Input: dimensioned drawing with shaded views. Units: mm. Origin: part minimum x, y, z. A direction names the side the tool comes from. Coordinates: 2 decimals unless noted, no trailing zeros. Order: outer loops, then holes, each group sorted by start corner. A loop starts at its lowest first (then second) coordinate and runs counter-clockwise, first axis right, second up. Notation, with made-up numbers: M -11,42.25 L 10,42.25 A32 ccw 10,78.25 Z; hole C 57.5,27.5 d6. An arc over 180 degrees is marked long. Use CSV: the item, a comma, the result in double quotes. Start each with the question number.
1. Pull-direction query (Y, two-part tool) for the marked faces 5, 6, 7 and 8; classes: pulls with the +Y half, pulls with the -Y half, needs draft (parallel to the pull), parting line crosses it, or undercut.
2. First-contact query: P1, Ø1.5, axis at y = 14.5, z = 37.5, coming from the -X side; P2, Ø3, axis at y = 3, z = 35, coming from the +X side; P3, Ø5, axis at y = 12.5, z = 54.5, coming from the +X side. Flat tips, straight axial feed; report the tip coordinate or a pass-through.
3. Section query C-C on z = 19. Return the cut outline in (x, y).
4. Section query B-B on x = 21. Return the cut outline in (y, z).
5. Material intervals for line 1 (Y direction, x = 24, z = 43.5); line 2 (Z direction, x = 25, y = 16.75); line 3 (X direction, y = 9.5, z = 5.5), sorted ascending.
6. Section query D-D on y = 16. Return the cut outline in (x, z).
7. Set-up query: the marked faces 1, 2, 3 and 4. Return all of +Z, -Z, +X, -X, +Y, -Y with unobstructed straight access to the full face (end or side cutting, diameter ignored); none if empty.
8. Section query A-A on y = 8.25. Return the cut outline in (x, z), and give its area (3 significant figures).
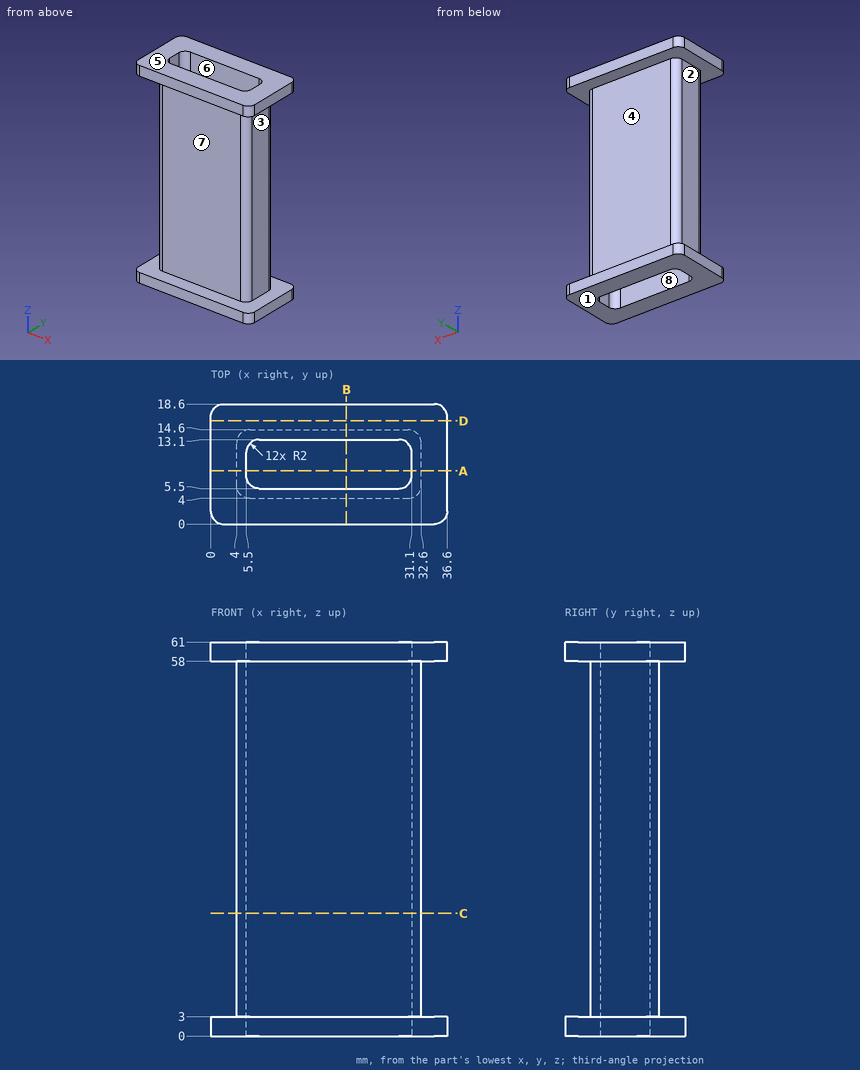
Results list:
1,face 5,"needs draft"
1,face 6,"undercut"
1,face 7,"pulls with the -Y half"
1,face 8,"undercut"
2,P1,"stops at x = 4.36"
2,P2,"stops at x = 31.92"
2,P3,"stops at x = 32.6"
3,outline,"M 4,6 A2 ccw 6,4 L 30.6,4 A2 ccw 32.6,6 L 32.6,12.6 A2 ccw 30.6,14.6 L 6,14.6 A2 ccw 4,12.6 Z; hole M 5.5,7.5 A2 ccw 7.5,5.5 L 29.1,5.5 A2 ccw 31.1,7.5 L 31.1,11.1 A2 ccw 29.1,13.1 L 7.5,13.1 A2 ccw 5.5,11.1 Z"
4,outline,"M 0,0 L 5.5,0 L 5.5,61 L 0,61 L 0,58 L 4,58 L 4,3 L 0,3 Z; M 13.1,0 L 18.6,0 L 18.6,3 L 14.6,3 L 14.6,58 L 18.6,58 L 18.6,61 L 13.1,61 Z"
5,line 1,"y = 4 to 5.5, 13.1 to 14.6"
5,line 2,"z = 0 to 3, 58 to 61"
5,line 3,"x = 4 to 5.5, 31.1 to 32.6"
6,outline,"M 0,0 L 36.6,0 L 36.6,3 L 0,3 Z; M 0,58 L 36.6,58 L 36.6,61 L 0,61 Z"
7,face 1,"-Z, +X, -X, +Y, -Y"
7,face 2,"-X, +Y, -Y"
7,face 3,"+X, +Y, -Y"
7,face 4,"+X, -X, +Y"
8,outline,"M 0,0 L 5.5,0 L 5.5,61 L 0,61 L 0,58 L 4,58 L 4,3 L 0,3 Z; M 31.1,0 L 36.6,0 L 36.6,3 L 32.6,3 L 32.6,58 L 36.6,58 L 36.6,61 L 31.1,61 Z"
8,area,"231 mm²"
